Geometry check sheet. Reference: the model listing, model coordinates, mm. A direction names the side the tool comes from. Coordinates: 2 decimals unless noted, no trailing zeros. Write each loop counter-clockwise with the first axis right and the second up, starting at its lowest first coordinate (ties: lowest second). Pieces come first, ordered by that corner, then holes. Notation, with made-up numbers: (67.5, 50.25) -> (121.5, 50.25) arc R24 ccw to (121.5, 81.25) -> close; hole circle Ø2 at (39.25, 65). An arc over 180 degrees is marked (long way). Answer in a Markdown table with one row per item. Add a question column.
Q1. Section check B-B, the plane z = 0. Record the boundary of the cut face in (x, y).
Q2. Gauge pin test, flat end, axial feed: P1, Ø5, axis at x = -3, z = -6, coming from the -Y side. Record the tip position at first contact, or that the pin passes through.
Q3. Tool access check on faces 4 (the face through (0, -7, -1)), 5 (the face through (25, 0, 0)). Record the directions out of +Z, -Z, +X, -X, +Y, -Y that give a thin tool (end or side, any length) a straight path to the whole face; none if there is none.
Q4. Thickness scan on line 1 (Y direction, x = -20.5, z = 2); line 2 (X direction, y = -7, z = 0.5). Record the ranges inside material, lowest first.
Q5. Release check for a two-part mould opening along X. For faces 1 (the face through (0, 5, 0)), 2 (the face through (-20, -7, 14)), 3 (the face through (-25, 0, 0)) record: pulls with the +X half, pulls with the -X half, needs draft (parallel to the pull), parting line crosses it, or undercut.
Q6. Section check C-C, the plane y = -7.5. Record the boundary of the cut face in (x, z).
Q7. Section check A-A, the plane x = 0. Record the boundary of the cut face in (y, z), and give its area (3 significant figures).
Q8. Section check D-D, the plane x = -20. Record the boundary of the cut face in (y, z), and give its area (3 significant figures).
```python
from build123d import *

# Parameters (mm, degrees)
F0_W          = 10
F0_H          = 40
F1_DEPTH      = 25
F1_DEPTH_BACK = 25
F2_R          = 1
F3_DEPTH      = 4


with BuildPart() as f1:
    # F0 (on Right) → F1 (new body, two sides)
    with BuildSketch(Plane.YZ) as f1_sk:
        Rectangle(F0_W, F0_H)
    extrude(amount=F1_DEPTH)
    extrude(f1_sk.sketch, amount=-F1_DEPTH_BACK)

    # F2 (on face) → F3 (join)
    with BuildSketch(Plane.XZ.offset(5)):
        Circle(F2_R)
        with Locations((-20, 15)):
            Circle(F2_R)
        with Locations((-20, -15)):
            Circle(F2_R)
        with Locations((20, -15)):
            Circle(F2_R)
        with Locations((20, 15)):
            Circle(F2_R)
    extrude(amount=F3_DEPTH)


solid = f1.part
```
Calculated:
| question | item | result |
|---|---|---|
| 1 | outline | (-25, -5) -> (-1, -5) -> (-1, -9) -> (1, -9) -> (1, -5) -> (25, -5) -> (25, 5) -> (-25, 5) -> close |
| 2 | P1 | stops at y = -5 |
| 3 | face 4 | -Y |
| 3 | face 5 | +Z, -Z, +X, +Y, -Y |
| 4 | line 1 | y = -5 to 5 |
| 4 | line 2 | x = -0.87 to 0.87 |
| 5 | face 1 | needs draft |
| 5 | face 2 | undercut |
| 5 | face 3 | pulls with the -X half |
| 6 | outline | circle Ø2 at (-20, -15); circle Ø2 at (-20, 15); circle Ø2 at (0, 0); circle Ø2 at (20, -15); circle Ø2 at (20, 15) |
| 7 | outline | (-9, -1) -> (-5, -1) -> (-5, -20) -> (5, -20) -> (5, 20) -> (-5, 20) -> (-5, 1) -> (-9, 1) -> close |
| 7 | area | 408 mm² |
| 8 | outline | (-9, -16) -> (-5, -16) -> (-5, -20) -> (5, -20) -> (5, 20) -> (-5, 20) -> (-5, 16) -> (-9, 16) -> (-9, 14) -> (-5, 14) -> (-5, -14) -> (-9, -14) -> close |
| 8 | area | 416 mm² |
